```python
from build123d import *

# Parameters (mm, degrees)
AUFSATZ_LINEAR_AUSTRAGEN1_DEPTH = 15
SKIZZE3_R                       = 18.45
SCHNITT_LINEAR_AUSTRAGEN1_DEPTH = 9
SKIZZE4_R                       = 1.65
SCHNITT_LINEAR_AUSTRAGEN2_DEPTH = 11


with BuildPart() as part:
    # Skizze1 → Aufsatz-Linear austragen1 (new, symmetric)
    with BuildSketch(Plane.XY):
        with BuildLine():
            ThreePointArc((25, 15.5), (0, 40.5), (-25, 15.5))
            Line((-25, 15.5), (-15, 15.5))
            ThreePointArc((-15, 15.5), (0, 30.5), (15, 15.5))
            Line((15, 15.5), (25, 15.5))
        make_face()
        with BuildLine():
            Line((-15, 15.5), (-25, 15.5))
            ThreePointArc((-25, 15.5), (0, -9.5), (25, 15.5))
            Line((25, 15.5), (15, 15.5))
            ThreePointArc((15, 15.5), (0, 0.5), (-15, 15.5))
        make_face()
        with BuildLine():
            Line((-25, 15.5), (-25, -15.5))
            Line((-25, -15.5), (25, -15.5))
            Line((25, -15.5), (25, 15.5))
            ThreePointArc((25, 15.5), (0, -9.5), (-25, 15.5))
        make_face()
    extrude(amount=AUFSATZ_LINEAR_AUSTRAGEN1_DEPTH, both=True)

    # Skizze3 → Schnitt-Linear austragen1 (cut)
    with BuildSketch(Plane.XY.offset(15)):
        with Locations((0, 15.5)):
            Circle(SKIZZE3_R)
    schnitt_linear_austragen1 = extrude(amount=-SCHNITT_LINEAR_AUSTRAGEN1_DEPTH, mode=Mode.SUBTRACT)

    # Spiegeln1: Schnitt-Linear austragen1 across plane
    add(schnitt_linear_austragen1.mirror(Plane.XY), mode=Mode.SUBTRACT)

    # Skizze4 → Schnitt-Linear austragen2 (cut)
    with BuildSketch(Plane.XZ.offset(15.5)):
        with Locations(Location((-17, 0, 0), (0, 0, 270))):
            Circle(SKIZZE4_R)
        with Locations(Location((-7, 0, 0), (0, 0, 270))):
            Circle(SKIZZE4_R)
        with Locations(Location((7, 0, 0), (0, 0, 90))):
            Circle(SKIZZE4_R)
        with Locations(Location((17, 0, 0), (0, 0, 90))):
            Circle(SKIZZE4_R)
    extrude(amount=-SCHNITT_LINEAR_AUSTRAGEN2_DEPTH, mode=Mode.SUBTRACT)


solid = part.part
```
Input: part model. Units: mm. Frame: model coordinates. A direction names the side the tool comes from. Coordinates: 2 decimals unless noted, no trailing zeros. Loops run counter-clockwise (first coordinate to the right, second up) from the corner with the lowest first, then second, coordinate; pieces in that order, holes last.
Q1. Mould query, pull axis Y, two halves, no side actions, for faces 6 (the flat face through (7, -4.5, 0)), 7 (the cylindrical face through (0.55, 40.494, 0.21)), 8 (the flat face through (0, 31, 6)), 9 (the flat face through (11, 0, 15)). Classes: +Y half, -Y half, draft (parallel to the pull), parting line (faces both ways), or undercut.
Results are:
face 6: -Y half
face 7: +Y half
face 8: undercut
face 9: draft
Q2. Set-up query: faces 1 (the flat face through (-25, 0, 0)), 2 (the flat face through (25, 0, 0)), 3 (the cylindrical face through (9.919, 31.057, -10.563)), 4 (the cylindrical face through (-8, -10.08, 1.31)), 5 (the cylindrical face through (9.919, 31.057, 10.563)). Return all of +Z, -Z, +X, -X, +Y, -Y with unobstructed straight access to the full face (end or side cutting, diameter ignored); none if empty.
Results are:
face 1: +Z, -Z, -X, +Y, -Y
face 2: +Z, -Z, +X, +Y, -Y
face 3: -Z
face 4: -Y
face 5: +Z
Q3. Line query: line 1 along X through (y, z) = (-8.25, 0); line 2 along Z through (x, y) = (17, -11); line 3 along Z through (x, y) = (4, 30). Output: solid intervals per line, ascending.
Results are:
line 1: x = -25 to -18.65, -15.35 to -8.65, -5.35 to 5.35, 8.65 to 15.35, 18.65 to 25
line 2: z = -15 to -1.65, 1.65 to 15
line 3: z = -6 to 6
Q4. Section A-A, the plane y = -10.5. Return the cut outline in (x, z).
Results are:
outline: (-25, -15) - (25, -15) - (25, 15) - (-25, 15) - close; hole circle Ø3.3 at (-17, 0); hole circle Ø3.3 at (-7, 0); hole circle Ø3.3 at (7, 0); hole circle Ø3.3 at (17, 0)
Q5. Contact query for flat-ended pins moving along their axis: pin 1 (4 mm diameter, centred on x = -7, z = 0, fed in from +Y); pin 2 (8 mm diameter, centred on x = 0.5, z = -10.5, fed in from +Y); pin 3 (6 mm diameter, centred on x = -12, z = -4.5, fed in from +Y). Output: stop coordinate, or through.
Results are:
pin 1: stops at y = 39.99
pin 2: stops at y = 40.5
pin 3: stops at y = 38.82
Q6. Section D-D, the plane x = 11. Return the cut outline in (y, z), and give its area (3 significant figures).
Results are:
outline: (-15.5, -15) - (0.69, -15) - (0.69, -6) - (5.3, -6) - (5.3, 6) - (0.69, 6) - (0.69, 15) - (-15.5, 15) - close; (25.7, -6) - (30.31, -6) - (30.31, -15) - (37.95, -15) - (37.95, 15) - (30.31, 15) - (30.31, 6) - (25.7, 6) - close
area: 826 mm2
Q7. Section B-B, the plane z = -13. Return the cut outline in (x, y).
Results are:
outline: (-25, -15.5) - (25, -15.5) - (25, 15.5) arc R25 ccw to (-25, 15.5) - close; hole circle Ø36.9 at (0, 15.5)
Q8. Section C-C, the plane y = 4.5. Return the cut outline in (x, z).
Results are:
outline: (-25, -15) - (-14.81, -15) - (-14.81, -6) - (-10.2, -6) - (-10.2, 6) - (-14.81, 6) - (-14.81, 15) - (-25, 15) - close; (10.2, -6) - (14.81, -6) - (14.81, -15) - (25, -15) - (25, 15) - (14.81, 15) - (14.81, 6) - (10.2, 6) - close
